Here's how the part is built. I have some questions about the finished solid (model axes, mm). Face numbers are marked on the shaded views. Give positions to 0.01 mm unless a question says otherwise; leave off trailing zeros. Loops run counter-clockwise (first coordinate to the right, second up) from the corner with the lowest first, then second, coordinate; pieces in that order, holes last.
Q1. Will this pin go through, and if not, where does the flat tip stop? P1, Ø12, axis at x = 4, z = -5, coming from the -Y side.
Q2. I need wall thicknesses on line 1 (Z direction, x = -21.5, y = -6); line 2 (X direction, y = 10.75, z = 14); line 3 (Z direction, x = 20, y = 8.75). Which ranges of each line are inside material? Lowest first, please.
Q3. If we section it at C-C (z = 16): Please give me the cut outline in (x, y), plus the area to 3 significant figures.
Q4. We'd pull the mould along Z, two halves only. Please class the marked faces 1, 2, 3 and 4: +Z half, -Z half, draft (parallel to the pull), parting line (faces both ways), or undercut.
Q5. If we section it at B-B (z = 0): Please give me the cut outline in (x, y), plus the area to 4 significant figures.
Q6. If we section it at D-D (y = 1.5): Please give me the cut outline in (x, z).
Q7. If we section it at A-A (x = 3.5): Please give me the cut outline in (y, z).
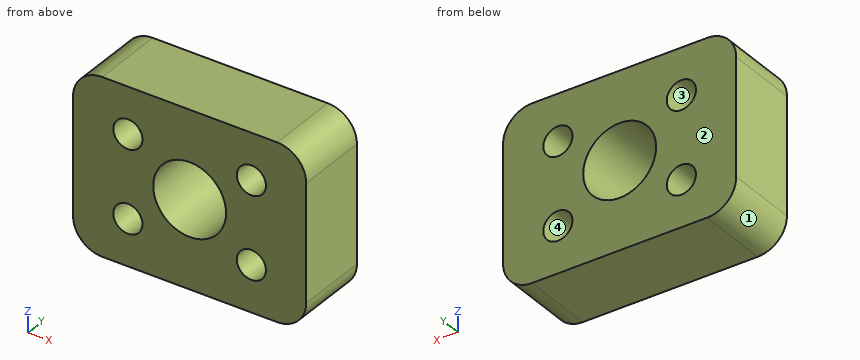
from build123d import *

# Parameters (mm, degrees)
F0_W     = 80
F0_H     = 60
F1_DEPTH = 12.5
F2_R     = 12.5
F3_DEPTH = 25
F4_R     = 10
F6_D     = 10


with BuildPart() as f1:
    # F0 (on Front) → F1 (new body, symmetric)
    with BuildSketch(Plane.XZ):
        Rectangle(F0_W, F0_H)
    extrude(amount=F1_DEPTH, both=True)

    # F2 (on face) → F3 (cut, through all)
    with BuildSketch(Plane.XZ.offset(12.5)):
        Circle(F2_R)
    extrude(amount=-F3_DEPTH, mode=Mode.SUBTRACT)

    # F4
    f4_edges = [f1.edges().sort_by_distance(p)[0] for p in [
        (-40, 0, 30),
        (40, 0, 30),
        (40, 0, -30),
        (-40, 0, -30),
    ]]
    fillet(f4_edges, radius=F4_R)

    # F6 (through all)
    with Locations(Plane.XZ.offset(12.5)):
        with Locations((-21.176471, 14.117647), (-21.176471, -14.117647), (21.176471, 14.117647), (21.176471, -14.117647)):
            Hole(F6_D / 2)


solid = f1.part
Check sheet entries:
1. P1: passes through
2. line 1: z = -30 to -19.11, -9.13 to 9.13, 19.11 to 30
2. line 2: x = -40 to -26.18, -16.18 to 16.18, 26.18 to 40
2. line 3: z = -30 to -18.98, -9.26 to 9.26, 18.98 to 30
3. outline: (-40, -12.5) - (-25.81, -12.5) - (-25.81, 12.5) - (-40, 12.5) - close; (-16.54, -12.5) - (16.54, -12.5) - (16.54, 12.5) - (-16.54, 12.5) - close; (25.81, -12.5) - (40, -12.5) - (40, 12.5) - (25.81, 12.5) - close
3. area: 1,540 mm2
4. face 1: -Z half
4. face 2: draft
4. face 3: undercut
4. face 4: undercut
5. outline: (-40, -12.5) - (-12.5, -12.5) - (-12.5, 12.5) - (-40, 12.5) - close; (12.5, -12.5) - (40, -12.5) - (40, 12.5) - (12.5, 12.5) - close
5. area: 1,375 mm2
6. outline: (-40, -20) arc R10 ccw to (-30, -30) - (30, -30) arc R10 ccw to (40, -20) - (40, 20) arc R10 ccw to (30, 30) - (-30, 30) arc R10 ccw to (-40, 20) - close; hole circle Ø10 at (-21.18, -14.12); hole circle Ø10 at (-21.18, 14.12); hole circle Ø25 at (0, 0); hole circle Ø10 at (21.18, -14.12); hole circle Ø10 at (21.18, 14.12)
7. outline: (-12.5, -30) - (12.5, -30) - (12.5, -12) - (-12.5, -12) - close; (-12.5, 12) - (12.5, 12) - (12.5, 30) - (-12.5, 30) - close
